Part model, mm, in its own coordinate system. Face numbers are marked on the shaded views. A direction names the side the tool comes from. Give positions to 0.01 mm unless a question says otherwise; leave off trailing zeros. Write each loop counter-clockwise with the first axis right and the second up, starting at its lowest first coordinate (ties: lowest second). Pieces come first, ordered by that corner, then holes. Notation, with made-up numbers: M 58,19 L 69,19 A14 cw 69,39 Z; hole C 23.25,-24.5 d8. An arc over 180 degrees is marked long. Answer as CSV lines item,"result". Start each with the question number.
1) Tool access for the marked faces 4, 5 and 6: list every direction of +Z, -Z, +X, -X, +Y, -Y with a clear straight run to the whole face (end or side of a thin tool).
2) Mould opens along Z. For the marked faces 1, 2 and 3 say: pulls with the +Z half, pulls with the -Z half, needs draft (parallel to the pull), parting line crosses it, or undercut.
3) Wall check: line 1 along Y through (x, z) = (-4, 13); line 2 along Z through (x, y) = (4.25, -10.5); line 3 along Y through (x, z) = (1.5, 12.75). Give the ranges that are in metal, low to high. Write a range as from..to.
4) Slice it at B-B, the plane y = 2.5. Give the cut face in (x, z), plus the area to 3 significant figures.
5) Slice it at A-A, the plane z = 7.5. Give the cut face in (x, y), plus the area to 3 significant figures.
6) Pin check, flat tips, straight feed: pin 1 Ø4 at (x, z) = (2, -32.5) entering from -Y; pin 2 Ø1.5 at (y, z) = (12.5, -23) entering from -X; pin 3 Ø2 at (y, z) = (17.5, 13) entering from +X. Stop position of each tip, or through.
```python
from build123d import *

# Parameters (mm, degrees)
SKETCH_1_W          = 15
SKETCH_1_H          = 44
EXTRUDE_1_DEPTH     = 8
SKETCH_10_R         = 3
SKETCH_10_R_2       = 2.5
CUT_EXTRUDE_1_DEPTH = 1
CUT_EXTRUDE_2_DEPTH = 2.6
SKETCH_12_R         = 2.5
SKETCH_12_R_2       = 2
CUT_EXTRUDE_3_DEPTH = 1
CUT_EXTRUDE_4_DEPTH = 2.5


with BuildPart() as part:
    # Sketch 1 → Extrude 1 (new body)
    with BuildSketch(Plane.XY.offset(9)):
        with Locations((1.5, 0)):
            Rectangle(SKETCH_1_W, SKETCH_1_H)
    extrude(amount=EXTRUDE_1_DEPTH)

    # Sketch 2 → Revolve 1 (revolve)
    with BuildSketch(Plane(origin=(0, 0, 0), x_dir=(0, 0, -1), z_dir=(1, 0, 0))):
        Polygon((-14, 10), (-14, 13), (35, 13), (35, 15), (40, 15), (40, 10), align=None)
    revolve(axis=Axis((0, 10, -40), (0, 0, 1)))

    # Sketch 3 → Revolve 2 (revolve)
    with BuildSketch(Plane(origin=(0, 0, 0), x_dir=(0, 0, -1), z_dir=(1, 0, 0))):
        Polygon((-14, -10), (-14, -7), (35, -7), (35, -5), (40, -5), (40, -10), align=None)
    revolve(axis=Axis((0, -10, -40), (0, 0, 1)))

    # Sketch 4 → Cut-Revolve 1 (revolve, cut)
    with BuildSketch(Plane(origin=(1.5, 0, 0), x_dir=(0, 0, -1), z_dir=(1, 0, 0))):
        Polygon((-17, 17.5), (-17, 19.5), (-16.621, 19.121), (-9.379, 19.121), (-9, 19.5), (-9, 17.5), align=None)
    revolve(axis=Axis((1.5, 17.5, 9), (0, 0, 1)), mode=Mode.SUBTRACT)

    # Sketch 5 → Cut-Revolve 2 (revolve, cut)
    with BuildSketch(Plane(origin=(1.5, 0, 0), x_dir=(0, 0, -1), z_dir=(1, 0, 0))):
        Polygon((-17, -17.5), (-17, -15.5), (-16.621, -15.879), (-9.379, -15.879), (-9, -15.5), (-9, -17.5), align=None)
    revolve(axis=Axis((1.5, -17.5, 9), (0, 0, 1)), mode=Mode.SUBTRACT)

    # Sketch 6 → Cut-Revolve 3 (revolve, cut)
    with BuildSketch(Plane.XY.offset(13)):
        Polygon((-6, 17.5), (-6, 19), (-5.7295, 18.7295), (-1, 18.7295), (-0.290147844, 17.5), align=None)
    revolve(axis=Axis((-0.290147844, 17.5, 13), (-1, 0, 0)), mode=Mode.SUBTRACT)

    # Sketch 7 → Cut-Revolve 4 (revolve, cut)
    with BuildSketch(Plane.XY.offset(13)):
        Polygon((-0.290147844, -17.5), (-1, -18.7295), (-5.7295, -18.7295), (-6, -19), (-6, -17.5), align=None)
    revolve(axis=Axis((-6, -17.5, 13), (1, 0, 0)), mode=Mode.SUBTRACT)

    # Sketch 8 → Cut-Revolve 5 (revolve, cut)
    with BuildSketch(Plane.XY.offset(13)):
        Polygon((3.290147844, 17.5), (4, 18.7295), (8.7295, 18.7295), (9, 19), (9, 17.5), align=None)
    revolve(axis=Axis((9, 17.5, 13), (-1, 0, 0)), mode=Mode.SUBTRACT)

    # Sketch 9 → Cut-Revolve 6 (revolve, cut)
    with BuildSketch(Plane.XY.offset(13)):
        Polygon((9, -17.5), (9, -19), (8.7295, -18.7295), (4, -18.7295), (3.290147844, -17.5), align=None)
    revolve(axis=Axis((3.290147844, -17.5, 13), (1, 0, 0)), mode=Mode.SUBTRACT)

    # Sketch 10 → Cut-Extrude 1 (cut)
    with BuildSketch(Plane.XY.offset(17)):
        with Locations((0, -10)):
            Circle(SKETCH_10_R)
        with Locations((0, -10)):
            Circle(SKETCH_10_R_2, mode=Mode.SUBTRACT)
    extrude(amount=-CUT_EXTRUDE_1_DEPTH, mode=Mode.SUBTRACT)

    # Sketch 11 → Cut-Extrude 2 (cut)
    with BuildSketch(Plane.XY.offset(17)):
        Polygon((-1.5011107, -10), (-0.75055535, -11.3), (0.75055535, -11.3), (1.5011107, -10), (0.75055535, -8.7), (-0.75055535, -8.7), align=None)
    extrude(amount=-CUT_EXTRUDE_2_DEPTH, mode=Mode.SUBTRACT)

    # Sketch 12 → Cut-Extrude 3 (cut)
    with BuildSketch(Plane(origin=(9, 0, 0), x_dir=(0, 0, -1), z_dir=(1, 0, 0))):
        with Locations((-13, 10)):
            Circle(SKETCH_12_R)
        with Locations((-13, 10)):
            Circle(SKETCH_12_R_2, mode=Mode.SUBTRACT)
    extrude(amount=-CUT_EXTRUDE_3_DEPTH, mode=Mode.SUBTRACT)

    # Sketch 13 → Cut-Extrude 4 (cut)
    with BuildSketch(Plane(origin=(9, 0, 0), x_dir=(0, 0, -1), z_dir=(1, 0, 0))):
        Polygon((-14.443375673, 10), (-13.721687836, 8.75), (-12.278312164, 8.75), (-11.556624327, 10), (-12.278312164, 11.25), (-13.721687836, 11.25), align=None)
    extrude(amount=-CUT_EXTRUDE_4_DEPTH, mode=Mode.SUBTRACT)


solid = part.part
```
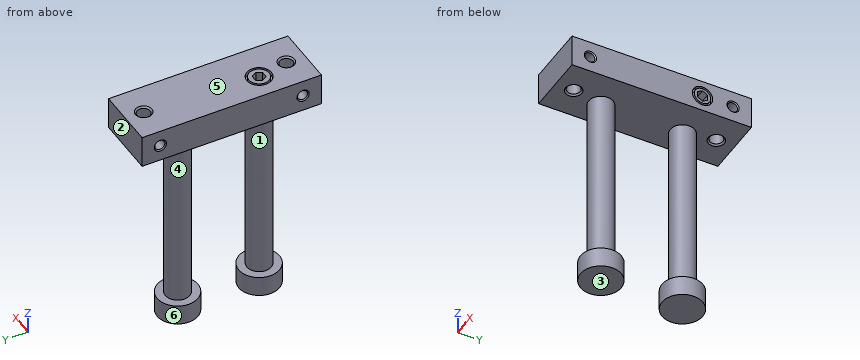
Found:
1,face 4,"none"
1,face 5,"+Z, +X, -X, +Y, -Y"
1,face 6,"-Z"
2,face 1,"undercut"
2,face 2,"needs draft"
2,face 3,"pulls with the -Z half"
3,line 1,"-22..-18.73, -16.27..16.27, 18.73..22"
3,line 2,"-40..-35, 9..17"
3,line 3,"-22..-19.12, -15.88..15.88, 19.12..22"
4,outline,"M -6,9 L 9,9 L 9,17 L -6,17 Z"
4,area,"120 mm²"
5,outline,"C 0,-10 d6; C 0,10 d6"
5,area,"56.5 mm²"
6,pin 1,"y = -13"
6,pin 2,"x = -2.44"
6,pin 3,"x = 3.87"
